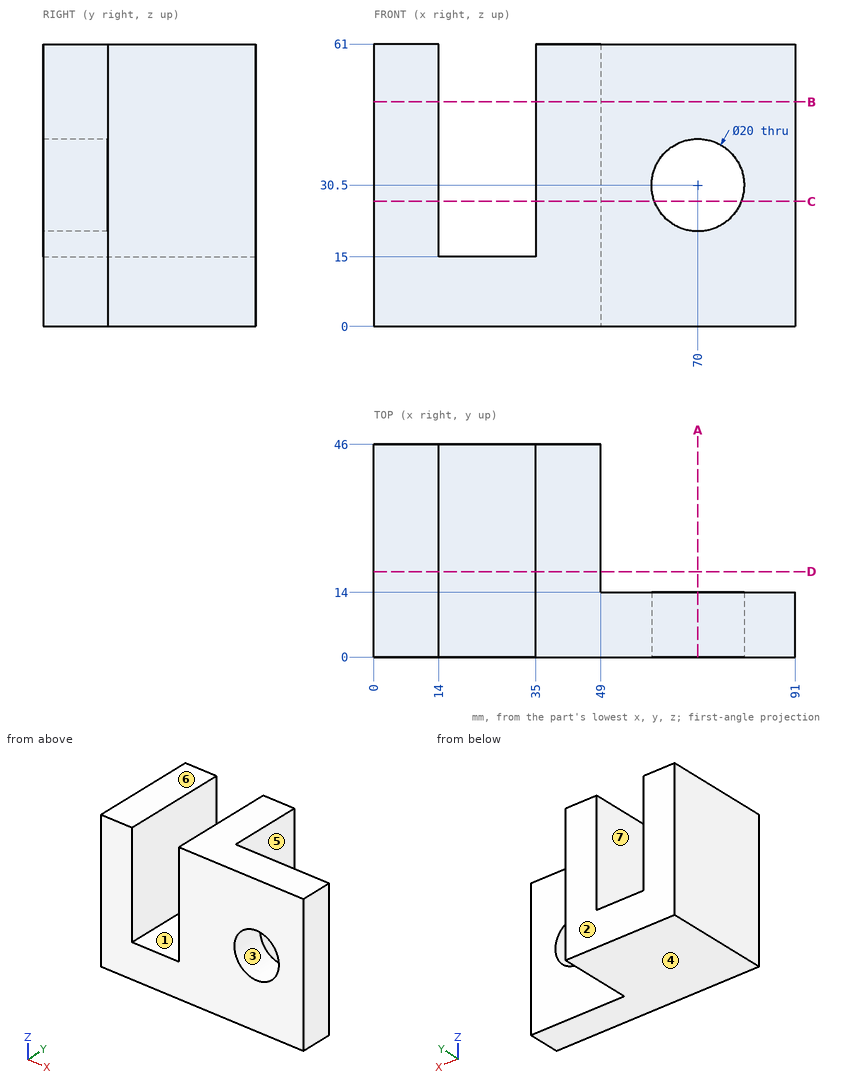
Geometry check sheet. Reference: drawing and pictorial views, mm from the part's lowest x, y, z. A direction names the side the tool comes from. Round coordinates to 2 decimals unless told otherwise and drop trailing zeros. Loops run counter-clockwise (first coordinate to the right, second up) from the corner with the lowest first, then second, coordinate; pieces in that order, holes last. Notation, with made-up numbers: (64, 29) - (89, 29) arc R14 cw to (89, 51) - close; hole circle Ø6 at (60.25, -35.75). An arc over 180 degrees is marked (long way). Answer in a Markdown table with one row per item. Add a question column.
Q1. Section check B-B on z = 48.5. Enter the section's corners in (x, y).
Q2. Section check C-C on z = 27. Enter the section's corners in (x, y), plus the area to 3 significant figures.
Q3. Gauge pin test, flat ends, axial feed: pin 1 (16 mm diameter, centred on y = 29, z = 45, fed in from +X); pin 2 (3 mm diameter, centred on x = 51, y = 26, fed in from -Z); pin 3 (5 mm diameter, centred on x = 74, z = 44, fed in from +Y); pin 4 (10.5 mm diameter, centred on x = 21.5, y = 29, fed in from +Z). Record the tip position at first contact, or that the pin passes through.
Q4. Material ranges on line 1 (X direction, y = 6.25, z = 30.5); line 2 (X direction, y = 27, z = 50.5); line 3 (Z direction, x = 16.5, y = 40), recorded low to high.
Q5. Tool access check on the marked faces 5, 6 and 7. Record the directions out of +Z, -Z, +X, -X, +Y, -Y that give a thin tool (end or side, any length) a straight path to the whole face; none if there is none.
Q6. Section check A-A on x = 70. Enter the section's corners in (y, z).
Q7. Release check for a two-part mould opening along Z. For the marked faces 1, 2, 3 and 4 record: pulls with the +Z half, pulls with the -Z half, needs draft (parallel to the pull), parting line crosses it, or undercut.
Q8. Section check D-D on y = 18.5. Enter the section's corners in (x, z), plus the area to 3 significant figures.
Found:
| question | item | result |
|---|---|---|
| 1 | outline | (0, 0) - (14, 0) - (14, 46) - (0, 46) - close; (35, 0) - (91, 0) - (91, 14) - (49, 14) - (49, 46) - (35, 46) - close |
| 2 | outline | (0, 0) - (14, 0) - (14, 46) - (0, 46) - close; (35, 0) - (60.63, 0) - (60.63, 14) - (49, 14) - (49, 46) - (35, 46) - close; (79.37, 0) - (91, 0) - (91, 14) - (79.37, 14) - close |
| 2 | area | 1,610 mm² |
| 3 | pin 1 | stops at x = 49 |
| 3 | pin 2 | passes through |
| 3 | pin 3 | stops at y = 14 |
| 3 | pin 4 | stops at z = 15 |
| 4 | line 1 | x = 0 to 14, 35 to 60, 80 to 91 |
| 4 | line 2 | x = 0 to 14, 35 to 49 |
| 4 | line 3 | z = 0 to 15 |
| 5 | face 5 | +Z, -Z, +X, +Y |
| 5 | face 6 | +Z, +X, -X, +Y, -Y |
| 5 | face 7 | +Z, +Y, -Y |
| 6 | outline | (0, 0) - (14, 0) - (14, 20.5) - (0, 20.5) - close; (0, 40.5) - (14, 40.5) - (14, 61) - (0, 61) - close |
| 7 | face 1 | pulls with the +Z half |
| 7 | face 2 | needs draft |
| 7 | face 3 | undercut |
| 7 | face 4 | pulls with the -Z half |
| 8 | outline | (0, 0) - (49, 0) - (49, 61) - (35, 61) - (35, 15) - (14, 15) - (14, 61) - (0, 61) - close |
| 8 | area | 2,020 mm² |
